Print and shaded views of the part. All mm, measured from the part's lowest x, y and z. Give positions to 0.01 mm unless a question says otherwise; leave off trailing zeros. Write each loop counter-clockwise with the first axis right and the second up, starting at its lowest first coordinate (ties: lowest second). Pieces come first, ordered by that corner, then holes.
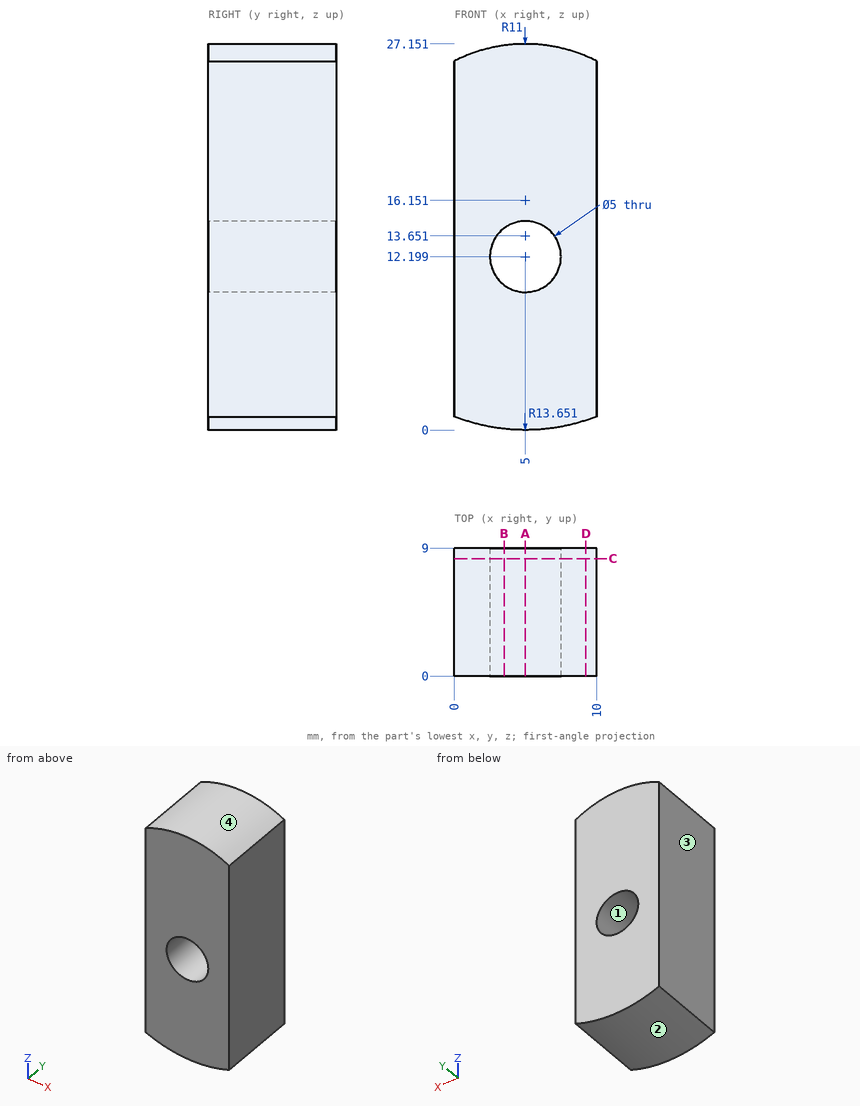
1. Mould opens along Z. For the marked faces 1, 2, 3 and 4 say: pulls with the +Z half, pulls with the -Z half, needs draft (parallel to the pull), parting line crosses it, or undercut.
2. Saw through at C-C on y = 8.25. Give the cut face in (x, z).
3. Saw through at B-B on x = 3.5. Give the cut face in (y, z).
4. Drop a flat-ended pin along its axis: pin 1 (4 mm diameter, centred on x = 1.5, y = 5.5, fed in from -Z). Give the stop position or say it passes through.
5. Saw through at D-D on x = 9.25. Give the cut face in (y, z).
6. Saw through at A-A on x = 5. Give the cut face in (y, z).
7. Drill centre lines: line 1 along X through (y, z) = (4.5, 12); line 2 along Z through (x, y) = (5.5, 5); line 3 along Z through (x, y) = (4, 3) (1 decimal). Where is each one in solid material? Low to high.
Outcome:
1. face 1: undercut
1. face 2: pulls with the -Z half
1. face 3: needs draft
1. face 4: pulls with the +Z half
2. outline: (0, 0.95) arc R13.65 ccw to (10, 0.95) - (10, 25.95) arc R11 ccw to (0, 25.95) - close; hole circle Ø5 at (5, 12.2)
3. outline: (0, 0.08) - (9, 0.08) - (9, 10.2) - (0, 10.2) - close; (0, 14.2) - (9, 14.2) - (9, 27.05) - (0, 27.05) - close
4. pin 1: stops at z = 0.08
5. outline: (0, 0.68) - (9, 0.68) - (9, 26.3) - (0, 26.3) - close
6. outline: (0, 0) - (9, 0) - (9, 9.7) - (0, 9.7) - close; (0, 14.7) - (9, 14.7) - (9, 27.15) - (0, 27.15) - close
7. line 1: x = 0 to 2.51, 7.49 to 10
7. line 2: z = 0.01 to 9.75, 14.65 to 27.14
7. line 3: z = 0 to 9.9, 14.5 to 27.1
